Here's how the part is built. I have some questions about the finished solid (model axes, mm). Face numbers are marked on the shaded views. Give positions to 0.01 mm unless a question says otherwise; leave off trailing zeros. Write each loop counter-clockwise with the first axis right and the second up, starting at its lowest first coordinate (ties: lowest second). Pieces come first, ordered by that corner, then holes. Notation, with made-up numbers: (23.25, 52) - (39.25, 52) arc R31 ccw to (39.25, 91) - close; hole circle Ø3 at (81, -32). An arc over 180 degrees is marked (long way). Use a Markdown table: item, result.
```python
from build123d import *

# Parameters (mm, degrees)
SKETCH1_R           = 40
SKETCH1_R_2         = 30
BOSS_EXTRUDE1_DEPTH = 250
SKETCH2_W           = 87.3454085
SKETCH2_H           = 86.102689272
BOSS_EXTRUDE2_DEPTH = 25
SKETCH3_W           = 88.230119684
SKETCH3_H           = 87.397760064
SKETCH3_R           = 15.055192133
BOSS_EXTRUDE3_DEPTH = 21
SKETCH4_R           = 6.558948387
SKETCH4_R_2         = 4.836777433
BOSS_EXTRUDE4_DEPTH = 35
SKETCH5_R           = 3.463305275
BOSS_EXTRUDE5_DEPTH = 320
BOSS_EXTRUDE6_DEPTH = 11


with BuildPart() as part:
    # Sketch1 → Boss-Extrude1 (new body)
    with BuildSketch(Plane.XY):
        Circle(SKETCH1_R)
        Circle(SKETCH1_R_2, mode=Mode.SUBTRACT)
    extrude(amount=BOSS_EXTRUDE1_DEPTH)

    # Sketch2 → Boss-Extrude2 (add)
    with BuildSketch(Plane.XY.offset(250)):
        Rectangle(SKETCH2_W, SKETCH2_H)
    extrude(amount=BOSS_EXTRUDE2_DEPTH)

    # Sketch3 → Boss-Extrude3 (add)
    with BuildSketch(Plane(origin=(0, 0, 0), x_dir=(-1, 0, 0), z_dir=(0, 0, -1))):
        Rectangle(SKETCH3_W, SKETCH3_H)
        Circle(SKETCH3_R, mode=Mode.SUBTRACT)
    extrude(amount=BOSS_EXTRUDE3_DEPTH)

    # Sketch4 → Boss-Extrude4 (add)
    with BuildSketch(Plane(origin=(44.115059842, 0, 0), x_dir=(0, 0, -1), z_dir=(1, 0, 0))):
        with Locations(Location((9.33886413, 0, 0), (0, 0, 180))):
            Circle(SKETCH4_R)
        with Locations((9.33886413, 0)):
            Circle(SKETCH4_R_2, mode=Mode.SUBTRACT)
    extrude(amount=BOSS_EXTRUDE4_DEPTH)

    # Sketch5 → Boss-Extrude5 (add)
    with BuildSketch(Plane(origin=(0, 0, -21), x_dir=(-1, 0, 0), z_dir=(0, 0, -1))):
        with Locations((-37.317802409, 36.268502466)):
            Circle(SKETCH5_R)
        with Locations((35.79642007, 36.268502466)):
            Circle(SKETCH5_R)
        with Locations((35.79642007, -37.807749255)):
            Circle(SKETCH5_R)
        with Locations((-37.317802409, -37.807749255)):
            Circle(SKETCH5_R)
    extrude(amount=-BOSS_EXTRUDE5_DEPTH)

    # Sketch6 → Boss-Extrude6 (add)
    with BuildSketch(Plane.XY.offset(275)):
        Polygon((-30.267074755, 32.921442439), (-30.1331084, 39.383525962), (-35.662453716, 42.73058599), (-41.325765385, 39.615562494), (-41.45973174, 33.153478971), (-35.930386425, 29.806418943), align=None)
        Polygon((40.930579927, 31.363930691), (43.37167492, 36.944973688), (39.758897402, 41.849545463), (33.70502489, 41.173074242), (31.263929897, 35.592031245), (34.876707416, 30.68745947), align=None)
        Polygon((-29.350890947, -41.042634272), (-29.772162906, -33.843199803), (-36.217692029, -30.608314786), (-42.241949193, -34.572864239), (-41.820677234, -41.772298708), (-35.375148111, -45.007183725), align=None)
        Polygon((40.930579927, -43.698880032), (44.226060077, -37.624557535), (40.613282559, -31.733426758), (33.70502489, -31.916618479), (30.40954474, -37.990940976), (34.022322258, -43.882071753), align=None)
    extrude(amount=BOSS_EXTRUDE6_DEPTH)


solid = part.part
```
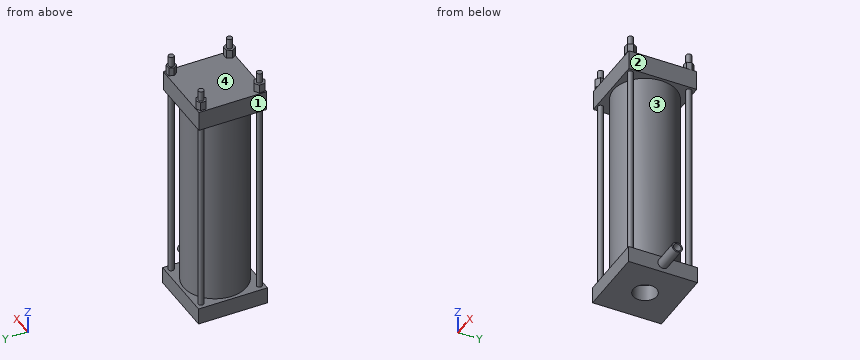
Item 1: If we section it at A-A, the plane y = 0: Write out the boundary of the cut face in (x, z).
Values:
| item | result |
|---|---|
| outline | (-44.12, -21) - (-15.06, -21) - (-15.06, 0) - (-30, 0) - (-30, 250) - (30, 250) - (30, 0) - (15.06, 0) - (15.06, -21) - (44.12, -21) - (44.12, -15.9) - (79.12, -15.9) - (79.12, -14.18) - (44.12, -14.18) - (44.12, -4.5) - (79.12, -4.5) - (79.12, -2.78) - (44.12, -2.78) - (44.12, 0) - (40, 0) - (40, 250) - (43.67, 250) - (43.67, 275) - (-43.67, 275) - (-43.67, 250) - (-40, 250) - (-40, 0) - (-44.12, 0) - close |
Item 2: If we section it at B-B, the plane z = 228: Write out the boundary of the cut face in (x, y).
Values:
| item | result |
|---|---|
| outline | circle Ø80 at (0, 0); circle Ø6.93 at (-35.8, -37.81); circle Ø6.93 at (-35.8, 36.27); circle Ø6.93 at (37.32, -37.81); circle Ø6.93 at (37.32, 36.27); hole circle Ø60 at (0, 0) |
Item 3: Thinking about a two-plate mould opening in X: for the marked faces 1, 2, 3 and 4, which applies, +X half, -X half, draft (parallel to the pull), parting line (faces both ways), or undercut?
Values:
| item | result |
|---|---|
| face 1 | -X half |
| face 2 | +X half |
| face 3 | undercut |
| face 4 | undercut |
Item 4: If we section it at C-C, the plane y = -18: Write out the boundary of the cut face in (x, z).
Values:
| item | result |
|---|---|
| outline | (-44.12, -21) - (44.12, -21) - (44.12, 0) - (35.72, 0) - (35.72, 250) - (43.67, 250) - (43.67, 275) - (-43.67, 275) - (-43.67, 250) - (-35.72, 250) - (-35.72, 0) - (-44.12, 0) - close; hole (-24, 0) - (24, 0) - (24, 250) - (-24, 250) - close |
Item 5: Will these pins go through, and if not, where does the flat tip stop? pin 1 Ø5 at (y, z) = (21, 148) entering from -X; pin 2 Ø4 at (y, z) = (14, 175) entering from -X; pin 3 Ø6 at (x, y) = (-11.5, 6.5) entering from +Z.
Values:
| item | result |
|---|---|
| pin 1 | stops at x = -35.46 |
| pin 2 | stops at x = -38.16 |
| pin 3 | stops at z = 275 |
Item 6: I need wall thicknesses on line 1 along Y through (x, z) = (0, -7); line 2 along Z through (x, y) = (63, -0.5); line 3 along Y through (x, z) = (0, 195). Which ranges of each line are inside material? Lowest first, please. Write a range as [from, to].
Values:
| item | result |
|---|---|
| line 1 | y = [-43.7, -15.06], [15.06, 43.7] |
| line 2 | z = [-15.88, -14.15], [-4.53, -2.8] |
| line 3 | y = [-40, -30], [30, 40] |
Item 7: If we section it at D-D, the plane x = 0: Write out the boundary of the cut face in (y, z).
Values:
| item | result |
|---|---|
| outline | (-43.7, -21) - (-15.06, -21) - (-15.06, 0) - (-30, 0) - (-30, 250) - (30, 250) - (30, 0) - (15.06, 0) - (15.06, -21) - (43.7, -21) - (43.7, 0) - (40, 0) - (40, 250) - (43.05, 250) - (43.05, 275) - (-43.05, 275) - (-43.05, 250) - (-40, 250) - (-40, 0) - (-43.7, 0) - close |
